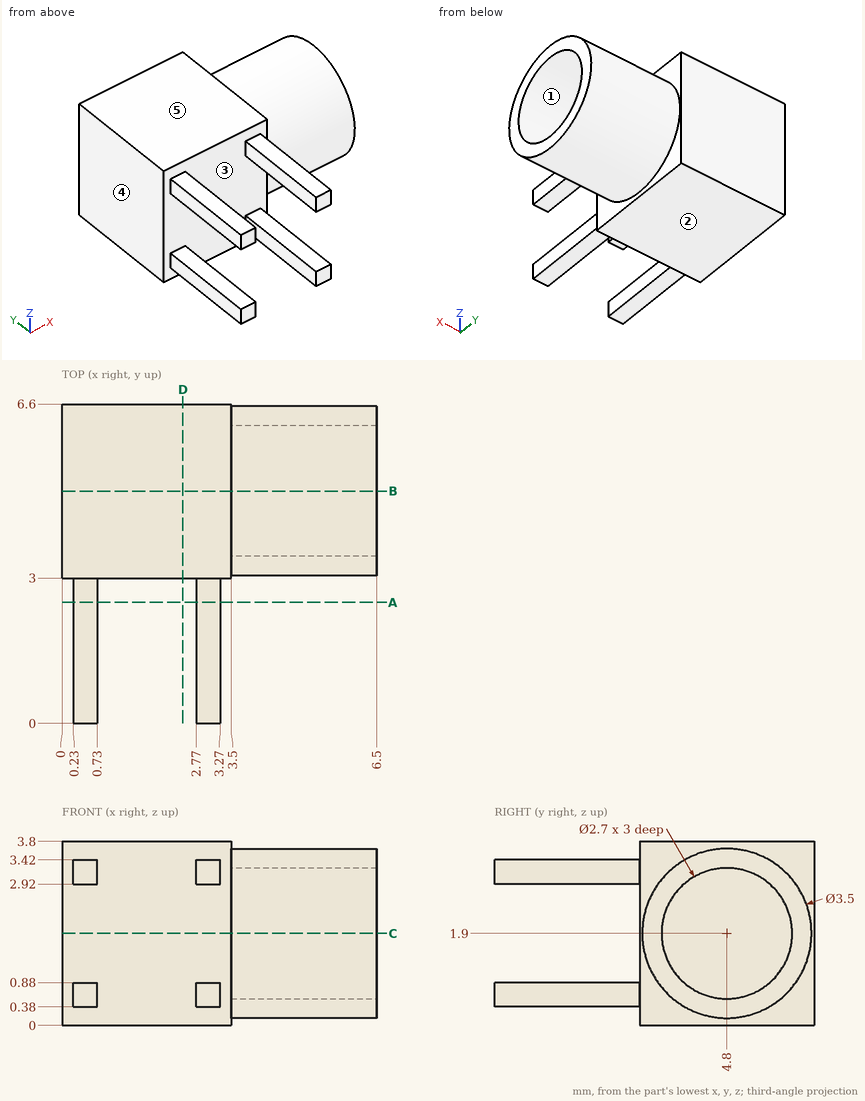
For this review, use the dimensioned drawing (mm, ordinates from the lowest corner) and the shaded views. A direction names the side the tool comes from. Coordinates: 2 decimals unless noted, no trailing zeros. Order: outer loops, then holes, each group sorted by start corner. A loop starts at its lowest first (then second) coordinate and runs counter-clockwise, first axis right, second up. Notation, with made-up numbers: (-31.5, 59.25) - (-15.5, 59.25) arc R22 ccw to (-15.5, 72.25) - close; hole circle Ø5 at (6, 55.25). An arc over 180 degrees is marked (long way). Answer as a JSON object with one key per item and string values. Group by question number.
1. For the marked faces 1 and 2, list the 3-axis set-ups (+Z, -Z, +X, -X, +Y, -Y) from which the entire face can be reached by the end or side of a thin tool; tool diameter is ignored.
2. We need section C-C on z = 1.9. State the section outline as (x, y) points.
3. We need section A-A on y = 2.5. State the section outline as (x, z) points, then the cut area to 3 significant figures.
4. We need section D-D on x = 2.5. State the section outline as (y, z) points.
5. The part is to be moulded in two halves that separate along X. For the marked faces 3, 4 and 5, say which applies: pulls with the +X half, pulls with the -X half, needs draft (parallel to the pull), parting line crosses it, or undercut.
6. We need section B-B on y = 4.8. State the section outline as (x, z) points, then the cut area to 3 significant figures.
7. For probe 1 along Z at (x, y) = (3, 1.5); probe 2 along Y at (x, z) = (5.3, 1.9); probe 3 along X at (y, z) = (1.25, 0.7), list the stretches that pass through material, from the lowest coordinate up.
8. Clearance check with flat-ended pins moving along their axes: P1, Ø0.6, axis at y = 1.5, z = 0.5, coming from the -X side; P2, Ø0.6, axis at y = 1, z = 3, coming from the +X side. State where each tip first meets the part, or that it passes through.
Final values:
{
 "1": {"face 1": "+X", "face 2": "-Z, +X, -X, +Y, -Y"},
 "2": {"outline": "(0, 3) - (3.5, 3) - (3.5, 3.05) - (6.5, 3.05) - (6.5, 3.45) - (3.5, 3.45) - (3.5, 6.15) - (6.5, 6.15) - (6.5, 6.55) - (3.5, 6.55) - (3.5, 6.6) - (0, 6.6) - close"},
 "3": {"outline": "(0.23, 0.38) - (0.73, 0.38) - (0.73, 0.88) - (0.23, 0.88) - close; (0.23, 2.92) - (0.73, 2.92) - (0.73, 3.42) - (0.23, 3.42) - close; (2.77, 0.38) - (3.27, 0.38) - (3.27, 0.88) - (2.77, 0.88) - close; (2.77, 2.92) - (3.27, 2.92) - (3.27, 3.42) - (2.77, 3.42) - close", "area": "1.00 mm²"},
 "4": {"outline": "(3, 0) - (6.6, 0) - (6.6, 3.8) - (3, 3.8) - close"},
 "5": {"face 3": "undercut", "face 4": "pulls with the -X half", "face 5": "needs draft"},
 "6": {"outline": "(0, 0) - (3.5, 0) - (3.5, 0.15) - (6.5, 0.15) - (6.5, 0.55) - (3.5, 0.55) - (3.5, 3.25) - (6.5, 3.25) - (6.5, 3.65) - (3.5, 3.65) - (3.5, 3.8) - (0, 3.8) - close", "area": "15.7 mm²"},
 "7": {"probe 1": "0.38 to 0.88, 2.92 to 3.42", "probe 2": "3.05 to 3.45, 6.15 to 6.55", "probe 3": "0.23 to 0.73, 2.77 to 3.27"},
 "8": {"P1": "x = 0.23", "P2": "x = 3.27"}
}
